from build123d import *

# Parameters (mm, degrees)
SKETCH1_W           = 350
SKETCH1_H           = 56.2
BOSS_EXTRUDE1_DEPTH = 10
SKETCH2_W           = 56.2
SKETCH2_H           = 56.2
CUT_EXTRUDE1_DEPTH  = 5
SKETCH3_W           = 10
SKETCH3_H           = 56.2
BOSS_EXTRUDE2_DEPTH = 10
SKETCH4_W           = 10
SKETCH4_H           = 56.2
BOSS_EXTRUDE3_DEPTH = 10
CUT_EXTRUDE2_DEPTH  = 56.2
SKETCH6_W           = 10
SKETCH6_H           = 56.2
BOSS_EXTRUDE4_DEPTH = 10
SKETCH7_W           = 10
SKETCH7_H           = 56.2
BOSS_EXTRUDE5_DEPTH = 10
CUT_EXTRUDE3_DEPTH  = 56.2
SKETCH9_W           = 30
SKETCH9_H           = 30
CUT_EXTRUDE4_DEPTH  = 5
SKETCH10_R          = 3
CUT_EXTRUDE5_DEPTH  = 5
SKETCH11_W          = 2.5
SKETCH11_H          = 15
CUT_EXTRUDE6_DEPTH  = 7
SKETCH12_W          = 2.5
SKETCH12_H          = 15
CUT_EXTRUDE7_DEPTH  = 7
SKETCH14_W          = 279.3
SKETCH14_H          = 56.2
CUT_EXTRUDE10_DEPTH = 10
SKETCH15_W          = 20
SKETCH15_H          = 56.2
CUT_EXTRUDE11_DEPTH = 10


with BuildPart() as part:
    # Sketch1 → Boss-Extrude1 (new body)
    with BuildSketch(Plane.XY):
        Rectangle(SKETCH1_W, SKETCH1_H)
    extrude(amount=BOSS_EXTRUDE1_DEPTH)

    # Sketch2 → Cut-Extrude1 (cut)
    with BuildSketch(Plane.XY.offset(10)):
        Rectangle(SKETCH2_W, SKETCH2_H)
    extrude(amount=-CUT_EXTRUDE1_DEPTH, mode=Mode.SUBTRACT)

    # Sketch3 → Boss-Extrude2 (add)
    with BuildSketch(Plane(origin=(175, 0, 0), x_dir=(0, 0, -1), z_dir=(1, 0, 0))):
        with Locations((-5, 0)):
            Rectangle(SKETCH3_W, SKETCH3_H)
    extrude(amount=BOSS_EXTRUDE2_DEPTH)

    # Sketch4 → Boss-Extrude3 (add)
    with BuildSketch(Plane.XY.offset(10)):
        with Locations((180, 0)):
            Rectangle(SKETCH4_W, SKETCH4_H)
    extrude(amount=BOSS_EXTRUDE3_DEPTH)

    # Sketch5 → Cut-Extrude2 (cut)
    with BuildSketch(Plane(origin=(0, 28.1, 0), x_dir=(1, 0, 0), z_dir=(0, 1, 0))):
        Polygon((175, -20), (185, -10), (185, -20), align=None)
    extrude(amount=-CUT_EXTRUDE2_DEPTH, mode=Mode.SUBTRACT)

    # Sketch6 → Boss-Extrude4 (add)
    with BuildSketch(Plane.ZY.offset(175)):
        with Locations((5, 0)):
            Rectangle(SKETCH6_W, SKETCH6_H)
    extrude(amount=BOSS_EXTRUDE4_DEPTH)

    # Sketch7 → Boss-Extrude5 (add)
    with BuildSketch(Plane.XY.offset(10)):
        with Locations((-180, 0)):
            Rectangle(SKETCH7_W, SKETCH7_H)
    extrude(amount=BOSS_EXTRUDE5_DEPTH)

    # Sketch8 → Cut-Extrude3 (cut)
    with BuildSketch(Plane(origin=(0, 28.1, 0), x_dir=(1, 0, 0), z_dir=(0, 1, 0))):
        Polygon((-175, -20), (-185, -10), (-185, -20), align=None)
    extrude(amount=-CUT_EXTRUDE3_DEPTH, mode=Mode.SUBTRACT)

    # Sketch9 → Cut-Extrude4 (cut)
    with BuildSketch(Plane.XY.offset(5)):
        Rectangle(SKETCH9_W, SKETCH9_H)
    extrude(amount=-CUT_EXTRUDE4_DEPTH, mode=Mode.SUBTRACT)

    # Sketch10 → Cut-Extrude5 (cut)
    with BuildSketch(Plane.XY.offset(5)):
        with Locations((21.55, 21.55)):
            Circle(SKETCH10_R)
        with Locations((-21.55, -21.55)):
            Circle(SKETCH10_R)
        with Locations((-21.55, 21.55)):
            Circle(SKETCH10_R)
        with Locations((21.55, -21.55)):
            Circle(SKETCH10_R)
    extrude(amount=-CUT_EXTRUDE5_DEPTH, mode=Mode.SUBTRACT)

    # Sketch11 → Cut-Extrude6 (cut)
    with BuildSketch(Plane(origin=(97.5, 0, 97.5), x_dir=(0.7071067811865478, 0, -0.7071067811865472), z_dir=(0.7071067811865472, 0, 0.7071067811865478))):
        with Locations((116.672618896, 0)):
            Rectangle(SKETCH11_W, SKETCH11_H)
    extrude(amount=-CUT_EXTRUDE6_DEPTH, mode=Mode.SUBTRACT)

    # Sketch12 → Cut-Extrude7 (cut)
    with BuildSketch(Plane(origin=(-97.5, 0, 97.5), x_dir=(0.7071067811865478, 0, 0.7071067811865472), z_dir=(-0.7071067811865472, 0, 0.7071067811865478))):
        with Locations((-116.672618896, 0)):
            Rectangle(SKETCH12_W, SKETCH12_H)
    extrude(amount=-CUT_EXTRUDE7_DEPTH, mode=Mode.SUBTRACT)

    # Sketch14 → Cut-Extrude10 (cut)
    with BuildSketch(Plane.XY.offset(10)):
        with Locations((45.35, 0)):
            Rectangle(SKETCH14_W, SKETCH14_H)
    extrude(amount=-CUT_EXTRUDE10_DEPTH, mode=Mode.SUBTRACT)


with BuildPart() as body_2:
    # of the pieces the cut leaves, the one that is kept (cut_extrude10_keep)
    add(part.part.solids().sort_by_distance((-185, -28.1, 0))[0])

    # Sketch15 → Cut-Extrude11 (cut)
    with BuildSketch(Plane.XY.offset(10)):
        with Locations((-104.3, 0)):
            Rectangle(SKETCH15_W, SKETCH15_H)
    extrude(amount=-CUT_EXTRUDE11_DEPTH, mode=Mode.SUBTRACT)


solid = body_2.part
Here's how the part is built. I have some questions about the finished solid (model axes, mm). A direction names the side the tool comes from. Coordinates: 2 decimals unless noted, no trailing zeros. Write each loop counter-clockwise with the first axis right and the second up, starting at its lowest first coordinate (ties: lowest second). Pieces come first, ordered by that corner, then holes.
Item 1: On a 3-axis mill with a long thin cutter (end or side, diameter ignored), from which of +Z, -Z, +X, -X, +Y, -Y can I reach the whole of each face in a straight line? I mean faces 1 (the flat face through (-179, 0, 16)), 2 (the flat face through (-175, 0, 15)), 3 (the flat face through (-178, 7.5, 13)). Say none if no direction works.
Item 2: Will these pins go through, and if not, where does the flat tip stop? pin 1 (6 mm diameter, centred on x = -156.5, y = 14, fed in from +Z); pin 2 (10 mm diameter, centred on y = -7.5, z = 17, fed in from -X); pin 3 (11 mm diameter, centred on y = 14, z = 17.5, fed in from +X).
Item 3: I want a section at B-B on x = -177. Write out the boundary of the cut face in (y, z).
Item 4: I want a section at C-C on y = 12.5. Write out the boundary of the cut face in (x, z).
Item 5: I want a section at A-A on y = -2.5. Write out the boundary of the cut face in (x, z).
Item 6: If we mould it in two halves opening along Y, with no side actions, what happens to faces 4 (the flat face through (-177.087, -0.105, 13.855)), 5 (the flat face through (-185, 0, 5)), 6 (the flat face through (-150, -28.1, 5)), 7 (the flat face through (-150, 28.1, 5))? For each: +Y half, -Y half, draft (parallel to the pull), parting line (faces both ways), or undercut.
Item 7: I want a section at D-D on z = 17.75. Write out the boundary of the cut face in (x, y), and give its area (3 significant figures).
Item 8: If I drill on line 1 (X direction, y = -5.5, z = 13); line 2 (Z direction, x = -174, y = -16.5); line 3 (Z direction, x = -175.5, y = -5.5), over which ranges is the centre line in solid material (lowest first)?
Findings below:
1. face 1: +Z, -X, +Y, -Y
1. face 2: +Z, +X, +Y, -Y
1. face 3: none
2. pin 1: stops at z = 10
2. pin 2: stops at x = -183
2. pin 3: stops at x = -175
3. outline: (-28.1, 0) - (28.1, 0) - (28.1, 18) - (-28.1, 18) - close; hole (-7.5, 10.23) - (7.5, 10.23) - (7.5, 13.77) - (-7.5, 13.77) - close
4. outline: (-185, 0) - (-114.3, 0) - (-114.3, 10) - (-175, 10) - (-175, 20) - (-185, 10) - close
5. outline: (-185, 0) - (-114.3, 0) - (-114.3, 10) - (-175, 10) - (-175, 10.1) - (-175.93, 9.17) - (-180.88, 14.12) - (-185, 10) - close; (-179.12, 15.88) - (-175, 11.77) - (-175, 20) - close
6. face 4: undercut
6. face 5: draft
6. face 6: -Y half
6. face 7: +Y half
7. outline: (-177.25, -28.1) - (-175, -28.1) - (-175, 28.1) - (-177.25, 28.1) - close
7. area: 126 mm2
8. line 1: x = -182 to -179.77, -176.23 to -175
8. line 2: z = 0 to 10
8. line 3: z = 0 to 9.6, 12.27 to 19.5
